Source: three-view drawing plus pictorial views. Frame: mm from the lowest corner of the part. Give positions to 0.01 mm unless a question says otherwise; leave off trailing zeros. Loops run counter-clockwise (first coordinate to the right, second up) from the corner with the lowest first, then second, coordinate; pieces in that order, holes last.
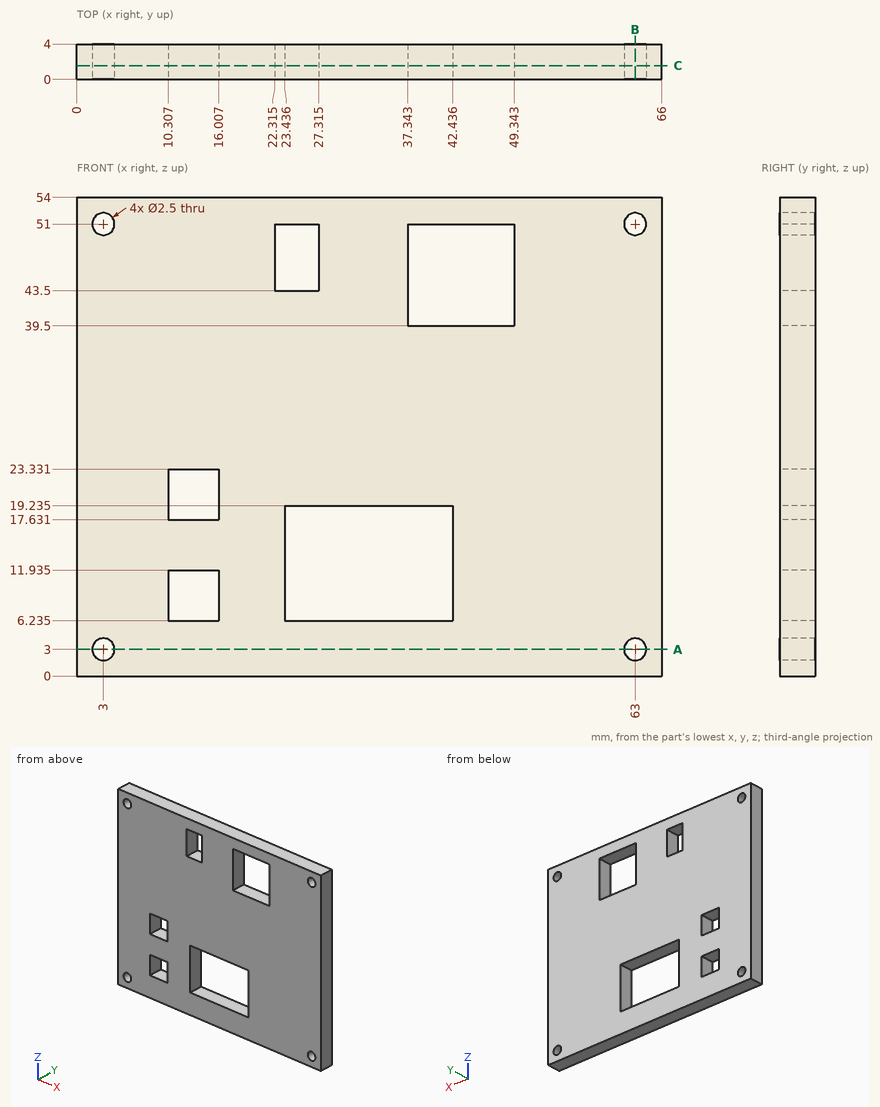
1) Contact query for a flat-ended pin moving along its axis: P1, Ø2, axis at x = 3, z = 51, coming from the -Y side. Output: stop coordinate, or through.
Checks:
P1: passes through
2) Cut plane B-B (x = 63). Return loops of the section in (y, z).
Checks:
outline: (0, 0) - (4, 0) - (4, 1.75) - (0, 1.75) - close; (0, 4.25) - (4, 4.25) - (4, 49.75) - (0, 49.75) - close; (0, 52.25) - (4, 52.25) - (4, 54) - (0, 54) - close
3) Ray query, probe 1 along Z at (x, y) = (3, 1.5); probe 2 along Z at (x, y) = (26, 0.55) (1 decimal); probe 3 along X at (y, z) = (3.3, 45.5) (1 decimal). Return the intervals inside material, ascending.
Checks:
probe 1: z = 0 to 1.75, 4.25 to 49.75, 52.25 to 54
probe 2: z = 0 to 6.2, 19.2 to 43.5, 51 to 54
probe 3: x = 0 to 22.3, 27.3 to 37.3, 49.3 to 66
4) Cut plane A-A (z = 3). Return loops of the section in (x, y).
Checks:
outline: (0, 0) - (1.75, 0) - (1.75, 4) - (0, 4) - close; (4.25, 0) - (61.75, 0) - (61.75, 4) - (4.25, 4) - close; (64.25, 0) - (66, 0) - (66, 4) - (64.25, 4) - close
5) Cut plane C-C (y = 1.55). State how many separate pieces and enclosed holes the cut face has, and give its area (3 significant figures).
Checks:
separate pieces: 1
enclosed holes: 9
area: 3,060 mm2
